For this review, take the finished solid that the model builds, in its own axes (mm). Give positions to 0.01 mm unless a question says otherwise; leave off trailing zeros. Write each loop counter-clockwise with the first axis right and the second up, starting at its lowest first coordinate (ties: lowest second). Pieces come first, ordered by that corner, then holes. Notation, with made-up numbers: M 36.25,2.25 L 61.25,2.25 A11 ccw 61.25,9.25 Z; hole C -25,53 d1. An arc over 180 degrees is marked long. Use one line per item in the form item = value. Start each with the question number.
Q1. Consider section B-B on z = 6.5. Write out the cut boundary in (x, y), and give its area (3 significant figures).
Q2. Consider section C-C on x = 0. Give the number of separate pieces and of enclosed holes in the cut face, and give its area (3 significant figures).
Q3. For probe 1 along X at (y, z) = (-0.85, -30); probe 2 along X at (y, z) = (1.4, 60); probe 3 along Y at (x, z) = (-6.5, 91.5), list the stretches that pass through material, from the lowest coordinate up. Write a range as [from, to].
Q4. Clearance check with a flat-ended pin moving along its axis: pin 1 Ø4.5 at (x, z) = (0, 60) entering from -Y. State where the tip first meets the part, or that it passes through.
```python
from build123d import *

# Parameters (mm, degrees)
SKETCH_1_W                   = 14
SKETCH_1_H                   = 200
EXTRUDE_1_DEPTH              = 5.2
CUT_EXTRUDE_1_DEPTH          = 201
CUT_EXTRUDE_2_DEPTH          = 201
CUT_EXTRUDE_3_DEPTH          = 201
CUT_EXTRUDE_4_DEPTH          = 201
HOLE_WIZARD_M3_1_D           = 3.5
HOLE_WIZARD_M3_1_DEPTH       = 5.2
HOLE_WIZARD_M3_1_CBORE_D     = 6
HOLE_WIZARD_M3_1_CBORE_DEPTH = 3.2
CHAMFER_1_SIZE               = 0.2475
FILLET_1_R                   = 0.14


with BuildPart() as part:
    # 草图1 → 凸台-拉伸1 (new body)
    with BuildSketch(Plane(origin=(0, 3.3, 0), x_dir=(1, 0, 0), z_dir=(0, 1, 0))):
        Rectangle(SKETCH_1_W, SKETCH_1_H)
    extrude(amount=-EXTRUDE_1_DEPTH)

    # 草图2 → 切除-拉伸1 (cut, through all)
    with BuildSketch(Plane(origin=(0, 0, -100), x_dir=(-1, 0, 0), z_dir=(0, 0, -1))):
        with BuildLine():
            Line((7, 1.23), (7, 2.44125))
            ThreePointArc((7, 2.44125), (6.766476308, 2.288808784), (6.593576466, 2.07))
            Line((6.593576466, 2.07), (5.893576466, 2.07))
            Line((5.893576466, 2.07), (5.893576466, 1.23))
            Line((5.893576466, 1.23), (7, 1.23))
        make_face()
    extrude(amount=-CUT_EXTRUDE_1_DEPTH, mode=Mode.SUBTRACT)

    # 草图3 → 切除-拉伸2 (cut, through all)
    with BuildSketch(Plane(origin=(0, 0, -100), x_dir=(-1, 0, 0), z_dir=(0, 0, -1))):
        with BuildLine():
            Line((7, 0.85875), (7, 1.23))
            Line((7, 1.23), (6.593576466, 1.23))
            ThreePointArc((6.593576466, 1.23), (6.766476308, 1.011191216), (7, 0.85875))
        make_face()
    extrude(amount=-CUT_EXTRUDE_2_DEPTH, mode=Mode.SUBTRACT)

    # 草图4 → 切除-拉伸3 (cut, through all)
    with BuildSketch(Plane(origin=(0, 0, -100), x_dir=(-1, 0, 0), z_dir=(0, 0, -1))):
        with BuildLine():
            Line((-7, 2.07), (-7, 0.85875))
            ThreePointArc((-7, 0.85875), (-6.766476308, 1.011191216), (-6.593576466, 1.23))
            Line((-6.593576466, 1.23), (-5.893576466, 1.23))
            Line((-5.893576466, 1.23), (-5.893576466, 2.07))
            Line((-5.893576466, 2.07), (-7, 2.07))
        make_face()
    extrude(amount=-CUT_EXTRUDE_3_DEPTH, mode=Mode.SUBTRACT)

    # 草图5 → 切除-拉伸4 (cut, through all)
    with BuildSketch(Plane(origin=(0, 0, -100), x_dir=(-1, 0, 0), z_dir=(0, 0, -1))):
        with BuildLine():
            Line((-7, 2.44125), (-7, 2.07))
            Line((-7, 2.07), (-6.593576466, 2.07))
            ThreePointArc((-6.593576466, 2.07), (-6.766476308, 2.288808784), (-7, 2.44125))
        make_face()
    extrude(amount=-CUT_EXTRUDE_4_DEPTH, mode=Mode.SUBTRACT)

    # M3 六角头机械螺钉的柱形沉头孔1
    with Locations(Plane(origin=(0, 3.3, 0), x_dir=(1, 0, 0), z_dir=(0, 1, 0))):
        with Locations((0, 90), (0, 60), (0, 30), (0, 0), (0, -30), (0, -60), (0, -90)):
            CounterBoreHole(HOLE_WIZARD_M3_1_D / 2, HOLE_WIZARD_M3_1_CBORE_D / 2, HOLE_WIZARD_M3_1_CBORE_DEPTH, depth=HOLE_WIZARD_M3_1_DEPTH)

    # 倒角1
    chamfer_1_edges = [part.edges().sort_by_distance(p)[0] for p in [
        (7, -1.9, 0),
        (-7, -1.9, 0),
        (7, 3.3, 0),
        (-7, 3.3, 0),
    ]]
    chamfer(chamfer_1_edges, length=CHAMFER_1_SIZE)

    # 圆角1
    fillet_1_edges = [part.edges().sort_by_distance(p)[0] for p in [
        (-5.893576466, 1.23, 0),
        (-5.893576466, 2.07, 0),
        (5.893576466, 2.07, 0),
        (5.893576466, 1.23, 0),
    ]]
    fillet(fillet_1_edges, radius=FILLET_1_R)


solid = part.part
```
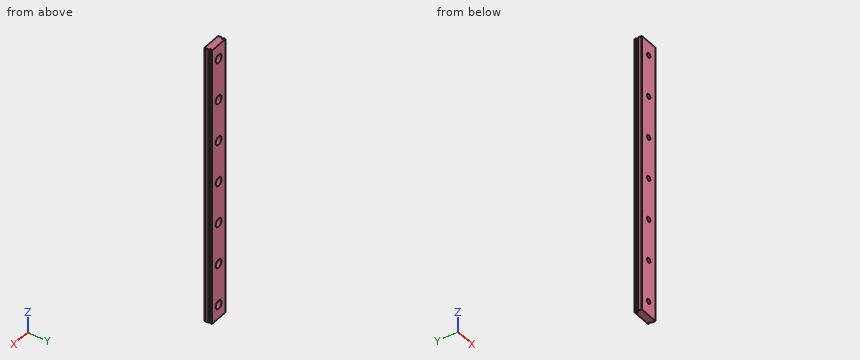
Working result:
q1.outline = M -7,-1.65 L -6.75,-1.9 L 6.75,-1.9 L 7,-1.65 L 7,0.86 A0.87 cw 6.59,1.23 L 6.03,1.23 A0.14 cw 5.89,1.37 L 5.89,1.93 A0.14 cw 6.03,2.07 L 6.59,2.07 A0.87 cw 7,2.44 L 7,3.05 L 6.75,3.3 L -6.75,3.3 L -7,3.05 L -7,2.44 A0.87 cw -6.59,2.07 L -6.03,2.07 A0.14 cw -5.89,1.93 L -5.89,1.37 A0.14 cw -6.03,1.23 L -6.59,1.23 A0.87 cw -7,0.86 Z
q1.area = 70.5 mm²
q2.separate_pieces = 8
q2.enclosed_holes = 0
q2.area = 857 mm²
q3.probe_1 = [-7, -1.75], [1.75, 7]
q3.probe_2 = [-5.89, -3], [3, 5.89]
q3.probe_3 = [-1.9, 1.23], [2.07, 3.3]
q4.pin_1 = -1.9
